Print and shaded views of the part. All mm, measured from the part's lowest x, y and z. Coordinates: 2 decimals unless noted, no trailing zeros. Loops run counter-clockwise (first coordinate to the right, second up) from the corner with the lowest first, then second, coordinate; pieces in that order, holes last.
1) Saw through at B-B, the plane z = 6.25. Write the cut outline in (x, y).
2) Saw through at A-A, the plane y = 39. Write the cut outline in (x, z).
3) Saw through at D-D, the plane x = 10. Write the cut outline in (y, z).
4) Wall check: line 1 along Y through (x, z) = (24, 0.5); line 2 along Y through (x, z) = (1.8, 3.25); line 3 along Y through (x, z) = (14, 1.5). Give the ranges that are in metal, low to high.
5) Saw through at C-C, the plane x = 1.8. Write the cut outline in (y, z).
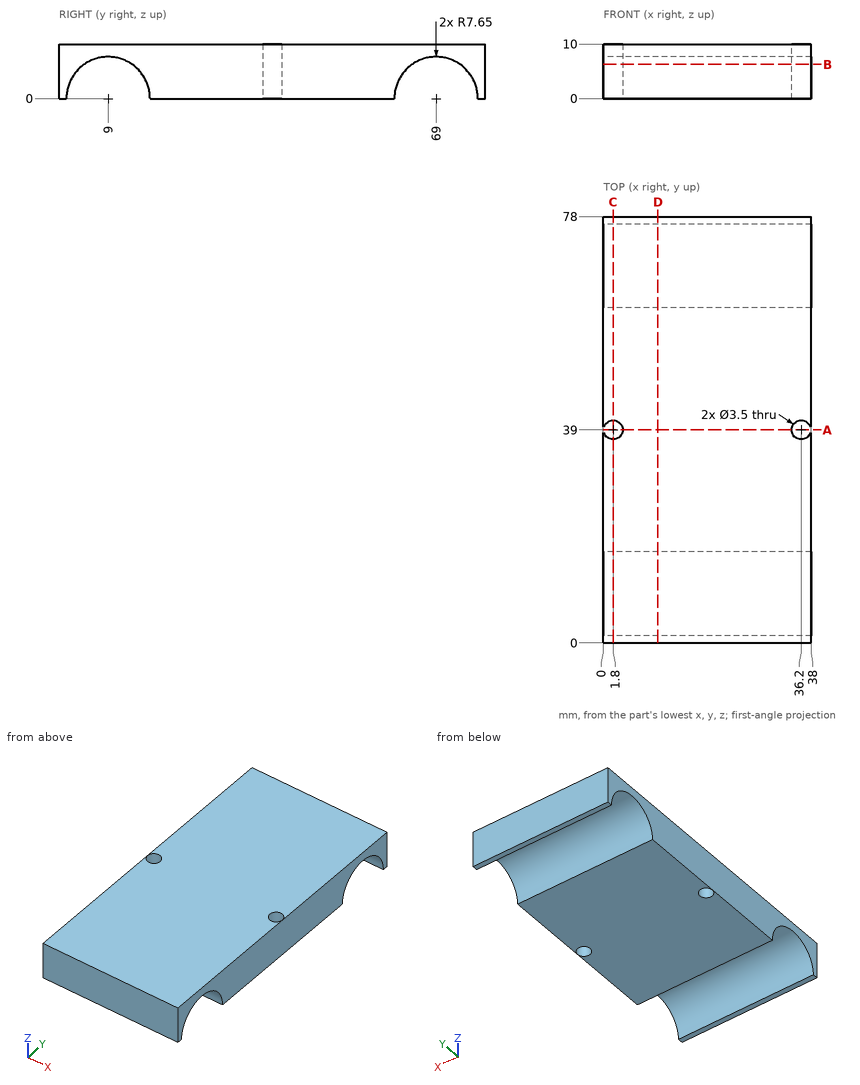
Data:
1. outline: (0, 0) - (38, 0) - (38, 4.59) - (0, 4.59) - close; (0, 13.41) - (38, 13.41) - (38, 64.59) - (0, 64.59) - close; (0, 73.41) - (38, 73.41) - (38, 78) - (0, 78) - close; hole circle Ø3.5 at (1.8, 39); hole circle Ø3.5 at (36.2, 39)
2. outline: (0, 0) - (0.05, 0) - (0.05, 10) - (0, 10) - close; (3.55, 0) - (34.45, 0) - (34.45, 10) - (3.55, 10) - close; (37.95, 0) - (38, 0) - (38, 10) - (37.95, 10) - close
3. outline: (0, 0) - (1.35, 0) arc R7.65 cw to (16.65, 0) - (61.35, 0) arc R7.65 cw to (76.65, 0) - (78, 0) - (78, 10) - (0, 10) - close
4. line 1: y = 0 to 1.37, 16.63 to 61.37, 76.63 to 78
4. line 2: y = 0 to 2.07, 15.93 to 37.25, 40.75 to 62.07, 75.93 to 78
4. line 3: y = 0 to 1.5, 16.5 to 61.5, 76.5 to 78
5. outline: (0, 0) - (1.35, 0) arc R7.65 cw to (16.65, 0) - (37.25, 0) - (37.25, 10) - (0, 10) - close; (40.75, 0) - (61.35, 0) arc R7.65 cw to (76.65, 0) - (78, 0) - (78, 10) - (40.75, 10) - close
